Autodesk Fusion 360 part; units mm, degrees
sketch "Sketch3" plane through (0, 0, 0) normal (0, 0, 1) x (1, 0, 0)
  line L0 (0, 0) -> (32, 0)
  line L1 (32, 0) -> (32, 32)
  line L2 (32, 32) -> (0, 32)
  line L3 (0, 32) -> (0, 0)
  line L4 (-0.5, 32.5) -> (-0.5, -0.5)
  line L5 (-0.5, -0.5) -> (32.5, -0.5)
  line L6 (32.5, -0.5) -> (32.5, 32.5)
  line L7 (32.5, 32.5) -> (-0.5, 32.5)
  line L8 (70, 32) -> (38, 32)
  line L9 (38, 32) -> (38, 0)
  line L10 (37.5, -0.5) -> (70.5, -0.5)
  line L11 (70.5, 32.5) -> (37.5, 32.5)
  line L12 (70, 0) -> (70, 32)
  line L13 (70.5, -0.5) -> (70.5, 32.5)
  line L14 (38, 0) -> (70, 0)
  line L15 (37.5, 32.5) -> (37.5, -0.5)
  line L16 (108, 32) -> (76, 32)
  line L17 (76, 32) -> (76, 0)
  line L18 (75.5, -0.5) -> (108.5, -0.5)
  line L19 (108.5, 32.5) -> (75.5, 32.5)
  line L20 (108, 0) -> (108, 32)
  line L21 (108.5, -0.5) -> (108.5, 32.5)
  line L22 (76, 0) -> (108, 0)
  line L23 (75.5, 32.5) -> (75.5, -0.5)
  line L24 (38, 32) -> (70, 0)
  line L25 (70, 32) -> (38, 0)
  line L26 (118, -10) -> (-10, -10)
  line L27 (-10, -10) -> (-10, 42)
  line L28 (-10, 42) -> (118, 42)
  line L29 (118, 42) -> (118, -10)
  line L30 (118, -10) -> (-10, 42) construction
  line L31 (-10, -10) -> (118, 42) construction
  circle A0 centre (3, 26) radius 2.05
  circle A1 centre (3, 26) radius 3.55
  circle A2 centre (29, 26) radius 3.55
  circle A3 centre (29, 26) radius 2.05
  circle A4 centre (29, 6) radius 2.05
  circle A5 centre (29, 6) radius 3.55
  circle A6 centre (3, 6) radius 2.05
  circle A7 centre (3, 6) radius 3.55
  circle A8 centre (67, 6) radius 2.05
  circle A9 centre (67, 6) radius 3.55
  circle A10 centre (41, 6) radius 2.05
  circle A11 centre (41, 6) radius 3.55
  circle A12 centre (67, 26) radius 2.05
  circle A13 centre (67, 26) radius 3.55
  circle A14 centre (41, 26) radius 2.05
  circle A15 centre (41, 26) radius 3.55
  circle A16 centre (105, 6) radius 2.05
  circle A17 centre (105, 6) radius 3.55
  circle A18 centre (79, 6) radius 2.05
  circle A19 centre (79, 6) radius 3.55
  circle A20 centre (105, 26) radius 2.05
  circle A21 centre (105, 26) radius 3.55
  circle A22 centre (79, 26) radius 2.05
  circle A23 centre (79, 26) radius 3.55
  line L32 (3, 22.45) -> (-0.5, 22.45)
  line L33 (-0.5, 22.45) -> (-0.5, 9.55)
  line L34 (-0.5, 9.55) -> (3, 9.55)
  line L35 (3, 9.55) -> (3, 22.45)
  line L36 (41, 22.45) -> (37.5, 22.45)
  line L37 (41, 9.55) -> (41, 22.45)
  line L38 (37.5, 9.55) -> (41, 9.55)
  line L39 (37.5, 22.45) -> (37.5, 9.55)
  line L40 (79, 22.45) -> (75.5, 22.45)
  line L41 (79, 9.55) -> (79, 22.45)
  line L42 (75.5, 9.55) -> (79, 9.55)
  line L43 (75.5, 22.45) -> (75.5, 9.55)
  circle A24 centre (-6, 38) radius 2.05
  circle A25 centre (-6, 38) radius 3.55
  circle A26 centre (54, 38) radius 2.05
  circle A27 centre (54, 38) radius 3.55
  circle A28 centre (114, 38) radius 2.05
  circle A29 centre (114, 38) radius 3.55
  circle A30 centre (-6, -6) radius 2.05
  circle A31 centre (-6, -6) radius 3.55
  circle A32 centre (54, -6) radius 2.05
  circle A33 centre (54, -6) radius 3.55
  circle A34 centre (114, -6) radius 2.05
  circle A35 centre (114, -6) radius 3.55
  point P0 (38, 0)
  point P1 (76, 0)
  point P2 (54, 16)
  dimension "d57" = 32
  dimension "d58" = 32
  dimension "d59" = 0.5
  dimension "d62" = 76
  dimension "d63" = 0
  dimension "d66" = 10
  dimension "d67" = 10
  dimension "d68" = 4.1
  dimension "d69" = 3
  dimension "d70" = 6
  dimension "d71" = 7.1
  dimension "d74" = 26
  dimension "d75" = 0
  dimension "d78" = 0
  dimension "d79" = -20
  dimension "d82" = 76
  dimension "d83" = 0
  dimension "d84" = 3.5
  dimension "d85" = 12.9
  dimension "d86" = 9.55
  dimension "d89" = 76
  dimension "d90" = 0
  dimension "d95" = 4
  dimension "d96" = 4
  dimension "d97" = 4.1
  dimension "d98" = 7.1
  dimension "d101" = 120
  dimension "d102" = 0
  dimension "d105" = 0
  dimension "d106" = -44
extrude "Extrude1" add sketch "Sketch3" along normal blind 1.5 contours L0 L1 L2 L3 A1 A2 A5 A7 L35 | L0 L1 L3 L4 L5 L6 A5 A7 | L3 L4 A7 | L3 A7 | L1 A5 | L1 L6 A5 | L3 L4 A7 L34 | L3 A7 L34 | L4 A7 | L1 L6 A2 A5 | L6 A5 | L1 A2 | L1 L6 A2 | L3 L4 A1 L32 | L3 A1 L32 | L3 A1 | L1 L2 L3 L4 L6 L7 A1 A2 | L6 A2 | L3 L4 A1 | L4 A1 | L8 L24 L25 A13 A15 | L8 L9 L11 L12 L13 L15 A13 A15 | L12 L25 A13 | L9 L24 A15 | L12 L13 A13 | L12 L25 A13 | L25 A13 | L9 L24 A15 | L9 L15 A15 | L24 A15 | L12 L13 A9 A13 | L12 L24 L25 A9 A13 | L13 A13 | L9 A15 L36 | L9 L15 A15 L36 | L15 A15 | L24 L25 A11 A15 L37 | L12 L13 A9 | L12 L24 A9 | L14 L24 L25 A9 A11 | L9 L10 L12 L13 L14 L15 A9 A11 | L12 L24 A9 | L13 A9 | L24 A9 | L25 A11 | L9 L25 A11 | L9 A11 L38 | L9 L15 A11 L38 | L9 L25 A11 | L9 L15 A11 | L15 A11 | L16 L17 L20 L22 A17 A19 A21 A23 L41 | L16 L17 L19 L20 L21 L23 A21 A23 | L20 L21 A21 | L20 A21 | L17 A23 | L17 L23 A23 | L20 L21 A17 A21 | L21 A21 | L17 A23 L40 | L17 L23 A23 L40 | L23 A23 | L20 L21 A17 | L20 A17 | L17 L18 L20 L21 L22 L23 A17 A19 | L21 A17 | L17 A19 L42 | L17 L23 A19 L42 | L17 A19 | L17 L23 A19 | L23 A19 | L26 L27 L28 L29 | A24 | A25 | A26 | A27 | A28 | A29 | A30 | A31 | A32 | A33 | A34 | A35
extrude "Extrude2" add sketch "Sketch3" along normal blind 3 contours L3 L4 A7 | L3 A7 | L1 A5 | L1 L6 A5 | L1 A2 | L1 L6 A2 | L3 A1 | L3 L4 A1 | L12 L13 A13 | L12 L25 A13 | L25 A13 | L9 L24 A15 | L9 L15 A15 | L24 A15 | L12 L13 A9 | L12 L24 A9 | L24 A9 | L25 A11 | L9 L25 A11 | L9 L15 A11 | L20 L21 A21 | L20 A21 | L17 A23 | L17 L23 A23 | L20 L21 A17 | L20 A17 | L17 A19 | L17 L23 A19 picked at (69.6833, 26) picked at (38.3167, 26) picked at (69.6833, 6) picked at (38.3167, 6)
extrude "Extrude3" add sketch "Sketch3" along normal blind 14 contours A25 | A27 | A29 | A31 | A33 | A35
fillet "Fillet1" radius 3.5 4 edges at (118, -10, 0.75) (-10, -10, 0.75) (118, 42, 0.75) (-10, 42, 0.75)
equation "d71 = d68 + 3 mm"
equation "d97 = d68"
equation "d98 = d97 + 3 mm"
equation "d111 = 3 mm + 12.5 mm - 1.5 mm"
Geometry check sheet. Reference: the model listing, model coordinates, mm. A direction names the side the tool comes from. Round coordinates to 2 decimals unless told otherwise and drop trailing zeros. Loops run counter-clockwise (first coordinate to the right, second up) from the corner with the lowest first, then second, coordinate; pieces in that order, holes last. Notation, with made-up numbers: (-36.75, 73.5) - (-13.75, 73.5) arc R31 ccw to (-13.75, 109.5) - close; hole circle Ø4 at (-25, -34). An arc over 180 degrees is marked (long way). Write each question's results on one line, items separated by ' | '. Start each with the question number.
Q1. Cross-section at C-C on x = 93. Enter the section's corners in (y, z).
Q2. Thickness scan on line 1 (Y direction, x = 54, z = 8.5); line 2 (Y direction, x = 78, z = 2.25); line 3 (X direction, y = -4.5, z = 11.25). Record the ranges inside material, lowest first. Write a range as [from, to].
Q3. Access from +Z, -Z, +X, -X, +Y, -Y to the whole of each face (thin tool, end or side, straight path). Record for faces 5 (the cylindrical face through (106.955, 25.384, 1.479)), 6 (the cylindrical face through (-6.77, -2.534, 7.662)).
Q4. Gauge pin test, flat ends, axial feed: P1, Ø4.5, axis at x = -6, y = 38, coming from the -Z side; P2, Ø3.5, axis at x = 67.5, y = 26, coming from the +Z side; P3, Ø2.5, axis at x = 3, y = 6, coming from the -Z side; P4, Ø0.6, axis at y = 26, z = 2, coming from the -X side. Record the tip position at first contact, or that the pin passes through.
Q5. Cross-section at B-B on x = 54. Enter the section's corners in (y, z), and give its area (3 significant figures).
Q6. Release check for a two-part mould opening along X. For faces 1 (the cylindrical face through (117, 40.95, 0.76)), 2 (the cylindrical face through (-6.77, 41.466, 7.662)), 3 (the cylindrical face through (-9, -8.95, 0.76)), 4 (the flat face through (30, 24, 3)) record: +X half, -X half, draft (parallel to the pull), parting line (faces both ways), or undercut.
Q7. Cross-section at A-A on z = 11.5. State how many separate pieces and enclosed holes the cut face has, and give its area (3 significant figures).
Answers below:
1) outline: (-10, 0) - (42, 0) - (42, 1.5) - (-10, 1.5) - close
2) line 1: y = [-9.55, -8.05], [-3.95, -2.45], [34.45, 35.95], [40.05, 41.55] | line 2: y = [2.59, 4.21], [7.79, 9.41], [22.59, 24.21], [27.79, 29.41] | line 3: x = [-9.22, -7.4], [-4.6, -2.78], [50.78, 52.6], [55.4, 57.22], [110.78, 112.6], [115.4, 117.22]
3) face 5: +Z, -Z | face 6: +Z
4) P1: stops at z = 0 | P2: stops at z = 3 | P3: passes through | P4: stops at x = -0.5
5) outline: (-10, 0) - (42, 0) - (42, 1.5) - (41.55, 1.5) - (41.55, 14) - (40.05, 14) - (40.05, 1.5) - (35.95, 1.5) - (35.95, 14) - (34.45, 14) - (34.45, 1.5) - (-2.45, 1.5) - (-2.45, 14) - (-3.95, 14) - (-3.95, 1.5) - (-8.05, 1.5) - (-8.05, 14) - (-9.55, 14) - (-9.55, 1.5) - (-10, 1.5) - close | area: 153 mm²
6) face 1: +X half | face 2: undercut | face 3: -X half | face 4: draft
7) separate pieces: 6 | enclosed holes: 6 | area: 158 mm²
